from build123d import *

# Parameters (mm, degrees)
SKETCH_1_R               = 12.2
EXTRUDE_1_DEPTH          = 50.8
SKETCH_2_R               = 2.75
EXTRUDE_2_DEPTH          = 4
SKETCH_4_R               = 6.5
EXTRUDE_3_DEPTH          = 2.6
SKETCH_5_R               = 3
EXTRUDE_4_DEPTH          = 2.9
EXTRUDE_START            = 11.5
SKETCH_6_R               = 2.75
EXTRUDE_5_DEPTH          = 11.5
CUT_EXTRUDE_1_DEPTH      = 11.5
CUT_EXTRUDE_1_DEPTH_BACK = 11.5
SKETCH_7_R               = 1.5
SKETCH_8_R               = 1.5
CUT_EXTRUDE_2_DEPTH      = 11.5


with BuildPart() as part:
    # Sketch 1 → Extrude 1 (new body)
    with BuildSketch(Plane(origin=(0, 0, 0), x_dir=(1, 0, 0), z_dir=(0, 1, 0))):
        with Locations(Location((0, 0, 0), (0, 0, 270))):
            Circle(SKETCH_1_R)
    extrude(amount=EXTRUDE_1_DEPTH)

    # Sketch 2 → Extrude 2 (add)
    with BuildSketch(Plane.XZ):
        with Locations(Location((0, 0, 0), (0, 0, 90))):
            Circle(SKETCH_2_R)
    extrude(amount=EXTRUDE_2_DEPTH)

    # Sketch 4 → Extrude 3 (add)
    with BuildSketch(Plane(origin=(0, 50.8, 0), x_dir=(1, 0, 0), z_dir=(0, 1, 0))):
        with Locations(Location((0, 0, 0), (0, 0, 270))):
            Circle(SKETCH_4_R)
    extrude(amount=EXTRUDE_3_DEPTH)

    # Sketch 5 → Extrude 4 (add)
    with BuildSketch(Plane(origin=(0, 53.4, 0), x_dir=(1, 0, 0), z_dir=(0, 1, 0))):
        with Locations(Location((0, 0, 0), (0, 0, 270))):
            Circle(SKETCH_5_R)
    extrude(amount=EXTRUDE_4_DEPTH)

    # Sketch 6 → Extrude 5 (add)
    with BuildSketch(Plane(origin=(0, 56.3, 0), x_dir=(1, 0, 0), z_dir=(0, 1, 0)).offset(EXTRUDE_START)):
        with Locations(Location((0, 0, 0), (0, 0, 270))):
            Circle(SKETCH_6_R)
    extrude(amount=-EXTRUDE_5_DEPTH)

    # Sketch 7 → Cut-Extrude 1 (cut, two sides: drawn at the far end of the back side and taken through both)
    with BuildSketch(Plane(origin=(0, 0, 0), x_dir=(0, 0, -1), z_dir=(1, 0, 0)).offset(-CUT_EXTRUDE_1_DEPTH_BACK)):
        with Locations(Location((0, 58.8, 0), (0, 0, 180))):
            Circle(SKETCH_7_R)
    extrude(amount=CUT_EXTRUDE_1_DEPTH + CUT_EXTRUDE_1_DEPTH_BACK, mode=Mode.SUBTRACT)

    # Sketch 8 → Cut-Extrude 2 (cut)
    with BuildSketch(Plane(origin=(0, 50.8, 0), x_dir=(1, 0, 0), z_dir=(0, 1, 0))):
        with Locations(Location((0, 9.5, 0), (0, 0, 270))):
            Circle(SKETCH_8_R)
        with Locations(Location((8.227241336, -4.75, 0), (0, 0, 270))):
            Circle(SKETCH_8_R)
        with Locations(Location((-8.227241336, -4.75, 0), (0, 0, 270))):
            Circle(SKETCH_8_R)
    extrude(amount=-CUT_EXTRUDE_2_DEPTH, mode=Mode.SUBTRACT)


solid = part.part
The listing builds one solid part. Answer for the finished solid, in the listing's coordinates (mm). A direction names the side the tool comes from. Coordinates: 2 decimals unless noted, no trailing zeros. Order: outer loops, then holes, each group sorted by start corner. A loop starts at its lowest first (then second) coordinate and runs counter-clockwise, first axis right, second up.
Q1. For a pull along X with two mould halves and no side action, classify faces 1 (the face through (8, 39.3, 5)), 2 (the face through (0.9, 54.83, 2.86)), 3 (the face through (-1, 53.4, 3)), 4 (the face through (0, 45, -11)) as pulls with the +X half, pulls with the -X half, needs draft (parallel to the pull), parting line crosses it, or undercut.
Q2. A cutting plane is placed at C-C, the plane y = 51.5. Write down the section's boundary in (x, z).
Q3. Which of the six approach directions +Z, -Z, +X, -X, +Y, -Y give full straight-line access (tool end or side, diameter ignored) to faces 5 (the face through (9.49, 45.13, 5.56)), 6 (the face through (0, -4, 0)), 7 (the face through (2.685, -1.972, -0.596))?
Q4. A cutting plane is placed at B-B, the plane x = 0. Write down the section's boundary in (y, z), and give its area (3 significant figures).
Q5. Consider line 1 (Z direction, x = -0.25, y = 58.8); line 2 (Y direction, x = 6.75, z = 2); line 3 (X direction, y = 42.25, z = 4.75). Determine where each line is inside the solid, lowest interval first.
Q6. Given P1, Ø2.5, axis at x = 8.23, z = 4.75, coming from the +Y side; P2, Ø6, axis at x = 8, z = -6.5, coming from the -Y side; P3, Ø3, axis at x = -5.5, y = 15, coming from the +Z side; P4, Ø2.5, axis at y = 58.8, z = 0, coming from the -X side (1 decimal), each flat-ended and moving along its own axis, determine where each tip first touches the part or whether it passes through.
Q7. A cutting plane is placed at A-A, the plane z = 0. Write down the section's boundary in (x, y), and give its area (3 significant figures).
Q8. A cutting plane is placed at D-D, the plane y = 58.8. Write down the section's boundary in (x, z).
Answers follow:
1. face 1: undercut
1. face 2: parting line crosses it
1. face 3: needs draft
1. face 4: undercut
2. outline: circle Ø13 at (0, 0)
3. face 5: +Y
3. face 6: +Z, -Z, +X, -X, -Y
3. face 7: -Y
4. outline: (-4, -2.75) - (0, -2.75) - (0, -12.2) - (50.8, -12.2) - (50.8, -11) - (39.3, -11) - (39.3, -8) - (50.8, -8) - (50.8, -6.5) - (53.4, -6.5) - (53.4, -3) - (56.3, -3) - (56.3, -2.75) - (67.8, -2.75) - (67.8, 2.75) - (56.3, 2.75) - (56.3, 3) - (53.4, 3) - (53.4, 6.5) - (50.8, 6.5) - (50.8, 12.2) - (0, 12.2) - (0, 2.75) - (-4, 2.75) - close; hole circle Ø3 at (58.8, 0)
4. area: 1,330 mm2
5. line 1: z = -2.74 to -1.5, 1.5 to 2.74
5. line 2: y = 0 to 50.8
5. line 3: x = -11.24 to -9.73, -6.73 to 6.73, 9.73 to 11.24
6. P1: stops at y = 39.3
6. P2: stops at y = 0
6. P3: stops at z = 11.53
6. P4: passes through
7. outline: (-12.2, 0) - (-2.75, 0) - (-2.75, -4) - (2.75, -4) - (2.75, 0) - (12.2, 0) - (12.2, 50.8) - (6.5, 50.8) - (6.5, 53.4) - (3, 53.4) - (3, 56.3) - (2.75, 56.3) - (2.75, 57.3) - (-2.75, 57.3) - (-2.75, 56.3) - (-3, 56.3) - (-3, 53.4) - (-6.5, 53.4) - (-6.5, 50.8) - (-12.2, 50.8) - close; (-2.75, 60.3) - (2.75, 60.3) - (2.75, 67.8) - (-2.75, 67.8) - close
7. area: 1,360 mm2
8. outline: (-2.3, -1.5) arc R2.75 ccw to (2.3, -1.5) - close; (-2.3, 1.5) - (2.3, 1.5) arc R2.75 ccw to start
